Read the model definition and answer for the solid it produces. Units are mm, in the model's axes. A direction names the side the tool comes from. Give positions to 0.01 mm unless a question says otherwise; leave off trailing zeros. Order: outer loops, then holes, each group sorted by start corner. A loop starts at its lowest first (then second) coordinate and runs counter-clockwise, first axis right, second up. Notation, with made-up numbers: (60.5, 63) -> (113.5, 63) arc R13 cw to (113.5, 71) -> close; hole circle Ø9 at (0, 46). An arc over 180 degrees is marked (long way). Answer as CSV lines item,"result". Start each with the question number.
1) For faces 1 (the face through (13.243, 11, 0)), 2 (the face through (16, 11, 1.75)), 3 (the face through (-4, 5, 1.25)), 4 (the face through (16, 24, -0.25)), 5 (the face through (16, 24, -5.25)), determine the directions among +Z, -Z, +X, -X, +Y, -Y from which every point of the face is accessible in a straight line to the end or side of a thin tool.
2) Find section C-C (z = 21). Determine the outline of the cut face in (x, y), and give its area (3 significant figures).
3) The mould has two halves that part along X. Classify faces 6 (the face through (16, 13, -3.75)), 7 (the face through (19.243, 11, 0)), 8 (the face through (-34, 4, 1.25)): +X half, -X half, draft (parallel to the pull), parting line (faces both ways), or undercut.
4) Find section B-B (x = 9.5). Determine the outline of the cut face in (y, z), and give its area (3 significant figures).
5) Straight lines are drawn through the part: L1, parallel to Z at x = 18.5, y = 9.5; L2, parallel to Y at x = 7, z = 26.5; L3, parallel to Z at x = 16, y = 23. For each, find the intervals that lie inside material, in ascending order. Write a range as from..to.
6) Flat-ended cylindrical pins translate along their axes: pin 1 Ø1.2 at (x, z) = (-34, 0.5) entering from +Y; pin 2 Ø6 at (x, y) = (-6.5, 10.5) entering from +Z; pin 3 Ø1.8 at (y, z) = (11.5, -6.5) entering from +X; pin 4 Ø1.5 at (x, y) = (-4, 6.5) entering from +Z. Find the tip coordinate at first contact, or state that the pin passes through.
7) Find section A-A (y = 20). Determine the outline of the cut face in (x, z).
```python
from build123d import *

# Parameters (mm, degrees)
SKETCH_1_W             = 100
SKETCH_1_H             = 100
EXTRUDE_1_DEPTH        = 1.5
EXTRUDE_1_DEPTH_BACK   = 20
SKETCH_2_R             = 0.75
EXTRUDE_2_DEPTH        = 0.75
SKETCH_3_W             = 1.5
SKETCH_3_H             = 3
EXTRUDE_3_DEPTH        = 1.5
SKETCH_5_W             = 3
SKETCH_5_H             = 1.5
EXTRUDE_4_DEPTH        = 3
SKETCH_7_R             = 0.75
EXTRUDE_5_DEPTH        = 2.5
SKETCH_8_W             = 6
SKETCH_8_H             = 9
EXTRUDE_6_DEPTH        = 10.4
SKETCH_9_W             = 3
SKETCH_9_H             = 1.5
EXTRUDE_7_DEPTH        = 4
SKETCH_10_R            = 0.75
EXTRUDE_8_DEPTH        = 3
SKETCH_11_W            = 6
SKETCH_11_H            = 2
CUT_EXTRUDE_1_DEPTH    = 10.4
SKETCH_12_W            = 6
SKETCH_12_H            = 3.5
EXTRUDE_9_DEPTH        = 20.17
SKETCH_13_W            = 3
SKETCH_13_H            = 1.5
EXTRUDE_10_DEPTH       = 4
SKETCH_14_R            = 0.75
EXTRUDE_11_DEPTH       = 2
PATTERN_LINEAR_2_COUNT = 2
PATTERN_LINEAR_2_PITCH = 13.6
SKETCH_16_W            = 6
SKETCH_16_H            = 8.75
CUT_EXTRUDE_2_DEPTH    = 9.25
SKETCH_17_W            = 6
SKETCH_17_H            = 2
CUT_EXTRUDE_3_DEPTH    = 1.65
SKETCH_18_W            = 3
SKETCH_18_H            = 1.5
EXTRUDE_12_DEPTH       = 4
SKETCH_19_R            = 0.75
EXTRUDE_13_DEPTH       = 3
EXTRUDE_14_DEPTH       = 1.5
SKETCH_21_W            = 0.75
SKETCH_21_H            = 3
CUT_EXTRUDE_4_DEPTH    = 1.5
SKETCH_22_W            = 1.5
SKETCH_22_H            = 0.5
EXTRUDE_15_DEPTH       = 2.5
SKETCH_23_W            = 3.5
SKETCH_23_H            = 14.4
CUT_EXTRUDE_5_DEPTH    = 6


with BuildPart() as part:
    # Sketch 1 → Extrude 1 (new body, two sides)
    with BuildSketch(Plane(origin=(0, 0, 0), x_dir=(1, 0, 0), z_dir=(0, 1, 0))) as extrude_1_sk:
        Rectangle(SKETCH_1_W, SKETCH_1_H)
    extrude(amount=EXTRUDE_1_DEPTH)
    extrude(extrude_1_sk.sketch, amount=-EXTRUDE_1_DEPTH_BACK)



with BuildPart() as body_2:
    # Sketch 2 → Extrude 2 (new body, symmetric)
    with BuildSketch(Plane.XY):
        with Locations((-40.336831864, 4.5)):
            Circle(SKETCH_2_R)
    extrude(amount=EXTRUDE_2_DEPTH, both=True)


with BuildPart() as part_1:
    add(part.part)

    add(body_2.part)  # Extrude 3 merges body 2
    # Sketch 3 → Extrude 3 (add)
    with BuildSketch(Plane.XY.offset(0.75)):
        with Locations((-40.336831864, 3)):
            Rectangle(SKETCH_3_W, SKETCH_3_H)
    extrude_3 = extrude(amount=EXTRUDE_3_DEPTH)

    # Mirror 1: Extrude 3 across plane
    add(extrude_3.mirror(Plane.XY))

    # Sketch 5 → Extrude 4 (add)
    with BuildSketch(Plane(origin=(0, 4.5, 0), x_dir=(1, 0, 0), z_dir=(0, 1, 0))):
        with Locations((-34.136831864, -0.5)):
            Rectangle(SKETCH_5_W, SKETCH_5_H)
        with Locations((-34.136831864, 3)):
            Rectangle(SKETCH_5_W, SKETCH_5_H)
    extrude(amount=-EXTRUDE_4_DEPTH)

    # Sketch 7 → Extrude 5 (add)
    with BuildSketch(Plane.XY.offset(-2.25)):
        with Locations((-34.136831864, 4.5)):
            Circle(SKETCH_7_R)
    extrude(amount=EXTRUDE_5_DEPTH)

    # Sketch 8 → Extrude 6 (add)
    with BuildSketch(Plane(origin=(0, 1.5, 0), x_dir=(1, 0, 0), z_dir=(0, 1, 0))):
        with Locations((-17.336831864, 1.25)):
            Rectangle(SKETCH_8_W, SKETCH_8_H)
    extrude_6 = extrude(amount=EXTRUDE_6_DEPTH)

    # Sketch 9 → Extrude 7 (add)
    with BuildSketch(Plane(origin=(0, 11.9, 0), x_dir=(1, 0, 0), z_dir=(0, 1, 0))):
        with Locations((-17.336831864, 3)):
            Rectangle(SKETCH_9_W, SKETCH_9_H)
        with Locations((-17.336831864, -0.5)):
            Rectangle(SKETCH_9_W, SKETCH_9_H)
    extrude(amount=EXTRUDE_7_DEPTH)

    # Sketch 10 → Extrude 8 (add)
    with BuildSketch(Plane.XY.offset(-2.25)):
        with Locations((-17.336831864, 14.9)):
            Circle(SKETCH_10_R)
    extrude(amount=EXTRUDE_8_DEPTH)

    # Sketch 11 → Cut-Extrude 1 (cut)
    with BuildSketch(Plane(origin=(0, 11.9, 0), x_dir=(1, 0, 0), z_dir=(0, 1, 0))):
        with Locations((-17.336831864, 1.25)):
            Rectangle(SKETCH_11_W, SKETCH_11_H)
    extrude(amount=-CUT_EXTRUDE_1_DEPTH, mode=Mode.SUBTRACT)

    # Sketch 12 → Extrude 9 (add)
    with BuildSketch(Plane(origin=(0, 1.5, 0), x_dir=(1, 0, 0), z_dir=(0, 1, 0))):
        with Locations((16.243168136, 0)):
            Rectangle(SKETCH_12_W, SKETCH_12_H)
        with Locations((16.243168136, 5.5)):
            Rectangle(SKETCH_12_W, SKETCH_12_H)
    extrude(amount=EXTRUDE_9_DEPTH)

    # Sketch 13 → Extrude 10 (add)
    with BuildSketch(Plane(origin=(0, 21.67, 0), x_dir=(1, 0, 0), z_dir=(0, 1, 0))):
        with Locations((16.243168136, 1)):
            Rectangle(SKETCH_13_W, SKETCH_13_H)
        with Locations((16.243168136, 4.5)):
            Rectangle(SKETCH_13_W, SKETCH_13_H)
    extrude(amount=EXTRUDE_10_DEPTH)

    # Sketch 14 → Extrude 11 (add)
    with BuildSketch(Plane.XY.offset(-3.75)):
        with Locations((16.243168136, 24.67)):
            Circle(SKETCH_14_R)
    extrude(amount=EXTRUDE_11_DEPTH)

    # Pattern Linear 2: Extrude 6 ×2
    with Locations(*[(i * PATTERN_LINEAR_2_PITCH, 0, 0) for i in range(1, PATTERN_LINEAR_2_COUNT)]):
        add(extrude_6)

    # Sketch 16 → Cut-Extrude 2 (cut, symmetric)
    with BuildSketch(Plane.XY):
        with Locations((-3.736831864, 7.525)):
            Rectangle(SKETCH_16_W, SKETCH_16_H)
    extrude(amount=CUT_EXTRUDE_2_DEPTH, both=True, mode=Mode.SUBTRACT)

    # Sketch 17 → Cut-Extrude 3 (cut)
    with BuildSketch(Plane(origin=(0, 3.15, 0), x_dir=(1, 0, 0), z_dir=(0, 1, 0))):
        with Locations((-3.736831864, 1.25)):
            Rectangle(SKETCH_17_W, SKETCH_17_H)
    extrude(amount=-CUT_EXTRUDE_3_DEPTH, mode=Mode.SUBTRACT)

    # Sketch 18 → Extrude 12 (add)
    with BuildSketch(Plane(origin=(0, 3.15, 0), x_dir=(1, 0, 0), z_dir=(0, 1, 0))):
        with Locations((-3.736831864, 3)):
            Rectangle(SKETCH_18_W, SKETCH_18_H)
        with Locations((-3.736831864, -0.5)):
            Rectangle(SKETCH_18_W, SKETCH_18_H)
    extrude(amount=EXTRUDE_12_DEPTH)

    # Sketch 19 → Extrude 13 (add)
    with BuildSketch(Plane.XY.offset(-2.25)):
        with Locations((-3.736831864, 6.15)):
            Circle(SKETCH_19_R)
    extrude(amount=EXTRUDE_13_DEPTH)

    # Sketch 20 → Extrude 14 (add)
    with BuildSketch(Plane(origin=(0, 4.5, 0), x_dir=(1, 0, 0), z_dir=(0, 1, 0))):
        Polygon((-32.636831864, 0.25), (-33.386831864, 0.25), (-33.386831864, -0.25), (-34.886831864, -0.25), (-34.886831864, 0.25), (-35.636831864, 0.25), (-35.636831864, -1.25), (-32.636831864, -1.25), align=None)
        Polygon((-35.636831864, 3.75), (-35.636831864, 2.25), (-34.886831864, 2.25), (-33.386831864, 2.25), (-32.636831864, 2.25), (-32.636831864, 3.75), align=None)
    extrude(amount=EXTRUDE_14_DEPTH)

    # Sketch 21 → Cut-Extrude 4 (cut)
    with BuildSketch(Plane.ZY.offset(41.086831864)):
        with Locations((1.875, 3)):
            Rectangle(SKETCH_21_W, SKETCH_21_H)
        with Locations((-1.875, 3)):
            Rectangle(SKETCH_21_W, SKETCH_21_H)
    extrude(amount=-CUT_EXTRUDE_4_DEPTH, mode=Mode.SUBTRACT)

    # Sketch 22 → Extrude 15 (add)
    with BuildSketch(Plane(origin=(0, 6, 0), x_dir=(1, 0, 0), z_dir=(0, 1, 0))):
        with Locations((-34.136831864, 0)):
            Rectangle(SKETCH_22_W, SKETCH_22_H)
    extrude(amount=-EXTRUDE_15_DEPTH)

    # Sketch 23 → Cut-Extrude 5 (cut)
    with BuildSketch(Plane.ZY.offset(20.336831864)):
        with Locations((-4, 8.7)):
            Rectangle(SKETCH_23_W, SKETCH_23_H)
    extrude(amount=-CUT_EXTRUDE_5_DEPTH, mode=Mode.SUBTRACT)


solid = part_1.part
```
Findings below:
1,face 1,"+Z, -Z, +Y"
1,face 2,"+Z, +X, +Y"
1,face 3,"+Z, +Y"
1,face 4,"+Z, +X, -X, +Y"
1,face 5,"-Z, +X, -X, +Y"
2,outline,"(-50, -20) -> (50, -20) -> (50, 1.5) -> (-50, 1.5) -> close"
2,area,"2,150 mm²"
3,face 6,"draft"
3,face 7,"+X half"
3,face 8,"undercut"
4,outline,"(-20, -50) -> (1.5, -50) -> (1.5, 50) -> (-20, 50) -> close"
4,area,"2,150 mm²"
5,L1,"-7.25..-3.75, -1.75..1.75"
5,L2,"-20..1.5"
5,L3,"-5.25..-3.75, -1.75..-0.25"
6,pin 1,"y = 6"
6,pin 2,"through"
6,pin 3,"x = 19.24"
6,pin 4,"z = 1.25"
7,outline,"(13.24, -7.25) -> (19.24, -7.25) -> (19.24, -3.75) -> (13.24, -3.75) -> close; (13.24, -1.75) -> (19.24, -1.75) -> (19.24, 1.75) -> (13.24, 1.75) -> close"
